```python
from build123d import *

# Parameters (mm, degrees)
SPESSORE1_T1 = 1
SMUSSO1_SIZE = 0.25


with BuildPart() as body_1:
    # Superficie-Rivoluzione1: a surface, the sketch's curves turned about an axis
    with BuildLine(Plane(origin=(0, 0, 0), x_dir=(0, 0, -1), z_dir=(1, 0, 0)), mode=Mode.PRIVATE) as superficie_rivoluzione1_1_path:
        Line((-9, 8.55), (-9, 11.5))
        Line((-9, 11.5), (-8, 12.5))
        Line((-8, 12.5), (8, 12.5))
        Line((8, 12.5), (9, 11.5))
        Line((9, 11.5), (9, 8.55))
    superficie_rivoluzione1_1 = Shell.revolve(superficie_rivoluzione1_1_path.wire(), 360, Axis((0, 0, 0), (0, 0, 1)))
    add(Solid.thicken(superficie_rivoluzione1_1, SPESSORE1_T1))

    # Smusso1
    smusso1_edges = [body_1.edges().sort_by_distance(p)[0] for p in [
        (0, -8.55, -9),
        (0, -8.55, 9),
    ]]
    chamfer(smusso1_edges, length=SMUSSO1_SIZE)


solid = body_1.part
```
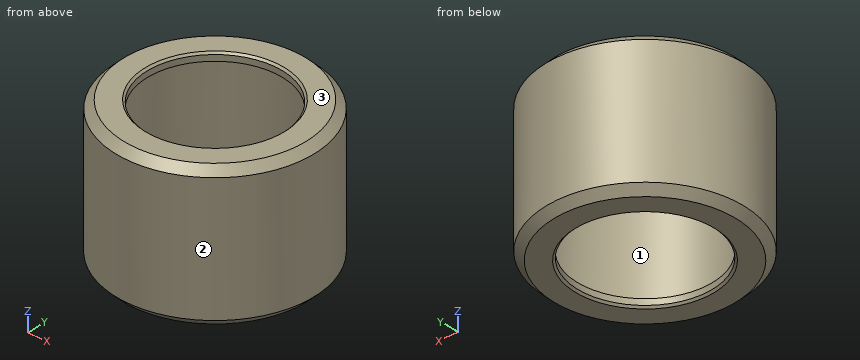
The model under review builds one solid part; all positions refer to its coordinate system, in mm. Face numbers are marked on the shaded views. Give positions to 0.01 mm unless a question says otherwise; leave off trailing zeros. Write each loop counter-clockwise with the first axis right and the second up, starting at its lowest first coordinate (ties: lowest second). Pieces come first, ordered by that corner, then holes. Notation, with made-up numbers: M 0,41 L 6,41 A25 ccw 6,69 Z; hole C 66.25,46 d4. An arc over 180 degrees is marked long. Write item = value, one per line. Start each with the question number.
Q1. We need section A-A (x = 0). State the section outline as (y, z) points, plus the area to 3 significant figures.
Q2. We need section C-C (z = -7). State the section outline as (x, y) points, plus the area to 3 significant figures.
Q3. Mouldability with a two-part tool opening along Z and no side actions: class the marked faces 1, 2 and 3 as released by +Z, released by -Z, zero draft, split by the parting line, or undercut.
Q4. For line 1 (Y direction, x = -6.25, z = -2); line 2 (Z direction, x = 1, y = 11); line 3 (X direction, y = 4.25, z = -0.5), list the stretches that pass through material, from the lowest coordinate up.
Q5. Clearance check with flat-ended pins moving along their axes: pin 1 (1 mm diameter, centred on y = 3, z = 4.5, fed in from -X); pin 2 (4 mm diameter, centred on x = 5.5, z = -3.5, fed in from +Y). State where each tip first meets the part, or that it passes through.
Result set:
q1.outline = M -12.5,-8 L -11.5,-9 L -8.8,-9 L -8.55,-8.75 L -8.55,-8 L -11.09,-8 L -11.5,-7.59 L -11.5,7.59 L -11.09,8 L -8.55,8 L -8.55,8.75 L -8.8,9 L -11.5,9 L -12.5,8 Z; M 8.55,-8.75 L 8.8,-9 L 11.5,-9 L 12.5,-8 L 12.5,8 L 11.5,9 L 8.8,9 L 8.55,8.75 L 8.55,8 L 11.09,8 L 11.5,7.59 L 11.5,-7.59 L 11.09,-8 L 8.55,-8 Z
q1.area = 46.0 mm2
q2.outline = C 0,0 d25; hole C 0,0 d23
q2.area = 75.4 mm2
q3.face_1 = undercut
q3.face_2 = zero draft
q3.face_3 = released by +Z
q4.line_1 = -10.83 to -9.65, 9.65 to 10.83
q4.line_2 = -9 to -8, 8 to 9
q4.line_3 = -11.76 to -10.69, 10.69 to 11.76
q5.pin_1 = -12.25
q5.pin_2 = 12
